Verification items for the finished model (mm, model axes). A direction names the side the tool comes from. Coordinates: 2 decimals unless noted, no trailing zeros. Order: outer loops, then holes, each group sorted by start corner. A loop starts at its lowest first (then second) coordinate and runs counter-clockwise, first axis right, second up. Notation, with made-up numbers: (-29, 19.5) -> (5, 19.5) arc R23 ccw to (5, 39.5) -> close; hole circle Ø2 at (22, -9.5). An arc over 180 degrees is marked (long way). Use CSV: the item, a comma, the result in double quotes. Start each with the question number.
1) Sectioned sample at D-D on z = 5.25. Record the boundary of the cut face in (x, y).
2) Tool access check on faces 4 (the cylindrical face through (1.412, -1.014, -4.483)), 5 (the flat face through (-6, 10.7, 9)), 6 (the flat face through (-6.2, 6, 0)). Record the directions out of +Z, -Z, +X, -X, +Y, -Y that give a thin tool (end or side, any length) a straight path to the whole face; none if there is none.
3) Go/stop test with flat-tipped pins: pin 1 (5 mm diameter, centred on y = 7, z = -10, fed in from -X); pin 2 (3 mm diameter, centred on x = 5, y = 1, fed in from +Z); pin 3 (6 mm diameter, centred on x = -1, z = 2, fed in from +Y). Record where each tip stops, or that it passes through.
4) Sectioned sample at C-C on y = 8.75. Record the boundary of the cut face in (x, z) (3 decimals), then the cut area to 3 significant figures.
5) Scan lines: line 1 along X through (y, z) = (-1, 0) (3 decimals); line 2 along X through (y, z) = (4, -5.5); line 3 along Y through (x, z) = (10.75, 5). Record each from-to range of solid material in increasing order.
6) Sectioned sample at A-A on z = 0. Record the boundary of the cut face in (x, y) (1 decimal).
7) Release check for a two-part mould opening along Z. For faces 1 (the cylindrical face through (3.991, 11.686, 12.674)), 2 (the flat face through (0, 6, -6.2)), 3 (the flat face through (2.3, -2, 4.4)) record: released by +Z, released by -Z, zero draft, split by the parting line, or undercut.
8) Sectioned sample at B-B on x = 0. Record the boundary of the cut face in (y, z) (1 decimal).
from build123d import *

# Parameters (mm, degrees)
SKETCH1_R           = 9.525
SKETCH1_W           = 12.4
SKETCH1_H           = 12.4
BOSS_EXTRUDE1_DEPTH = 12.70000008
BOSS_EXTRUDE3_START = -2
SKETCH2_R           = 13.2875
SKETCH2_R_2         = 9.525
BOSS_EXTRUDE3_DEPTH = 2
BOSS_EXTRUDE4_START = 2
SKETCH3_R           = 9.525
SKETCH3_R_2         = 4.7
BOSS_EXTRUDE4_DEPTH = 2


with BuildPart() as part:
    # Sketch1 → Boss-Extrude1 (new body)
    with BuildSketch(Plane(origin=(0, 0, 0), x_dir=(1, 0, 0), z_dir=(0, 1, 0))):
        with Locations(Location((0, 0, 0), (0, 0, 270))):
            Circle(SKETCH1_R)
        Rectangle(SKETCH1_W, SKETCH1_H, mode=Mode.SUBTRACT)
    extrude(amount=BOSS_EXTRUDE1_DEPTH)

    # Sketch2 → Boss-Extrude3 (add)
    with BuildSketch(Plane(origin=(0, 12.70000008, 0), x_dir=(1, 0, 0), z_dir=(0, 1, 0)).offset(BOSS_EXTRUDE3_START)):
        with Locations(Location((0, 0, 0), (0, 0, 270))):
            Circle(SKETCH2_R)
        with Locations(Location((0, 0, 0), (0, 0, 270))):
            Circle(SKETCH2_R_2, mode=Mode.SUBTRACT)
    extrude(amount=BOSS_EXTRUDE3_DEPTH)

    # Sketch3 → Boss-Extrude4 (add)
    with BuildSketch(Plane.XZ.offset(BOSS_EXTRUDE4_START)):
        with Locations(Location((0, 0, 0), (0, 0, 270))):
            Circle(SKETCH3_R)
        with Locations(Location((0, 0, 0), (0, 0, 270))):
            Circle(SKETCH3_R_2, mode=Mode.SUBTRACT)
    extrude(amount=-BOSS_EXTRUDE4_DEPTH)


solid = part.part
Answers follow:
1,outline,"(-12.21, 10.7) -> (-7.95, 10.7) -> (-7.95, -2) -> (7.95, -2) -> (7.95, 10.7) -> (12.21, 10.7) -> (12.21, 12.7) -> (6.2, 12.7) -> (6.2, 0) -> (-6.2, 0) -> (-6.2, 12.7) -> (-12.21, 12.7) -> close"
2,face 4,"+Y, -Y"
2,face 5,"-Y"
2,face 6,"+Y"
3,pin 1,"stops at x = -5.87"
3,pin 2,"stops at z = 8.86"
3,pin 3,"stops at y = 0"
4,outline,"circle Ø19.05 at (0, 0); hole (-6.2, -6.2) -> (6.2, -6.2) -> (6.2, 6.2) -> (-6.2, 6.2) -> close"
4,area,"131 mm²"
5,line 1,"x = -9.525 to -4.7, 4.7 to 9.525"
5,line 2,"x = -7.78 to -6.2, 6.2 to 7.78"
5,line 3,"y = 10.7 to 12.7"
6,outline,"(-13.3, 10.7) -> (-9.5, 10.7) -> (-9.5, -2) -> (-4.7, -2) -> (-4.7, 0) -> (-6.2, 0) -> (-6.2, 12.7) -> (-13.3, 12.7) -> close; (4.7, -2) -> (9.5, -2) -> (9.5, 10.7) -> (13.3, 10.7) -> (13.3, 12.7) -> (6.2, 12.7) -> (6.2, 0) -> (4.7, 0) -> close"
7,face 1,"split by the parting line"
7,face 2,"undercut"
7,face 3,"zero draft"
8,outline,"(-2, -9.5) -> (10.7, -9.5) -> (10.7, -13.3) -> (12.7, -13.3) -> (12.7, -6.2) -> (0, -6.2) -> (0, -4.7) -> (-2, -4.7) -> close; (-2, 4.7) -> (0, 4.7) -> (0, 6.2) -> (12.7, 6.2) -> (12.7, 13.3) -> (10.7, 13.3) -> (10.7, 9.5) -> (-2, 9.5) -> close"
